Read the model definition and answer for the solid it produces. Units are mm, in the model's axes. Coordinates: 2 decimals unless noted, no trailing zeros. Loops run counter-clockwise (first coordinate to the right, second up) from the corner with the lowest first, then second, coordinate; pieces in that order, holes last. Notation, with made-up numbers: (-29, -16) - (27, -16) arc R28 ccw to (27, 3) - close; hole circle Ø7 at (-15.5, -20). An arc over 180 degrees is marked (long way). Use one line per item in the form item = value. Start each with the question number.
1) A cutting plane is placed at C-C (z = 8.5). State how many separate pieces and enclosed holes the cut face has, and give its area (3 significant figures).
2) The mould has two halves that part along Y. Classify faces 1 (the face through (153.21, 173.15, 4.93)), 2 (the face through (221.595, -27.339, 5.07)), 3 (the face through (249.34, 0.04, 4.93)): released by +Y, released by -Y, zero draft, split by the parting line, or undercut.
3) Each of these flat-tipped pins is pushed along its axis until it touches: P1, Ø5, axis at y = -71, z = 7, coming from the -X side; P2, Ø5, axis at x = 8, z = 3, coming from the +Y side; P3, Ø5, axis at y = 136.5, z = 6, coming from the -X side; P4, Ø12, axis at x = 11, y = 127.5, coming from the +Z side. Where does it stop, or does it pass through?
4) Consider line 1 (Y direction, x = 0, z = 4); line 2 (X direction, y = 32, z = 4.5); line 3 (X direction, y = 155, z = 5.5). Determine where each line is inside the solid, lowest interval first.
5) A cutting plane is placed at A-A (x = -90). Give the vertices of the cut face in (y, z), and give its area (3 significant figures).
6) A cutting plane is placed at B-B (y = -139.5). Give the vertices of the cut face in (x, z), and give its area (3 significant figures).
from build123d import *

# Parameters (mm, degrees)
ESQUISSE1_R             = 47.5
BOSS_EXTRU_1_DEPTH      = 10
ESQUISSE9_W             = 150
ESQUISSE9_H             = 120
BOSS_EXTRU_2_DEPTH      = 10
ESQUISSE10_W            = 10
ESQUISSE10_H            = 50
ESQUISSE10_W_2          = 50
ESQUISSE10_H_2          = 10
ENL_V_MAT_EXTRU_1_DEPTH = 10


with BuildPart() as part:
    # Esquisse1 → Boss.-Extru.1 (new body)
    with BuildSketch(Plane.XY):
        Polygon((-255.775862069, 10.959681362), (-205, -75.190256718), (205, -75.190256718), (255.775862069, 10.959681362), (50, 336.353741833), (-50, 336.353741833), align=None)
        with Locations((-157.5, 0)):
            Circle(ESQUISSE1_R, mode=Mode.SUBTRACT)
        with Locations((-52.5, 0)):
            Circle(ESQUISSE1_R, mode=Mode.SUBTRACT)
        with Locations((52.5, 0)):
            Circle(ESQUISSE1_R, mode=Mode.SUBTRACT)
        with Locations((157.5, 0)):
            Circle(ESQUISSE1_R, mode=Mode.SUBTRACT)
        with Locations((-105, 90.932667397)):
            Circle(ESQUISSE1_R, mode=Mode.SUBTRACT)
        with Locations((0, 90.932667397)):
            Circle(ESQUISSE1_R, mode=Mode.SUBTRACT)
        with Locations((105, 90.932667397)):
            Circle(ESQUISSE1_R, mode=Mode.SUBTRACT)
        with Locations((-52.5, 181.865334795)):
            Circle(ESQUISSE1_R, mode=Mode.SUBTRACT)
        with Locations((52.5, 181.865334795)):
            Circle(ESQUISSE1_R, mode=Mode.SUBTRACT)
        with Locations((0, 272.798002192)):
            Circle(ESQUISSE1_R, mode=Mode.SUBTRACT)
    extrude(amount=BOSS_EXTRU_1_DEPTH)

    # Esquisse9 → Boss.-Extru.2 (add)
    with BuildSketch(Plane.XY.offset(10)):
        with Locations((0, -135.190256718)):
            Rectangle(ESQUISSE9_W, ESQUISSE9_H)
    extrude(amount=-BOSS_EXTRU_2_DEPTH)

    # Esquisse10 → Enlèv. mat.-Extru.1 (cut)
    with BuildSketch(Plane.XY.offset(10)):
        with Locations((-70, -129.244737692)):
            Rectangle(ESQUISSE10_W, ESQUISSE10_H)
        with Locations((0, -190.190256718)):
            Rectangle(ESQUISSE10_W_2, ESQUISSE10_H_2)
        with Locations((-140, -70.190256718)):
            Rectangle(ESQUISSE10_W_2, ESQUISSE10_H_2)
        Polygon((-217.693965517, -53.652772198), (-209.078971709, -48.575185991), (-234.466902744, -5.500216951), (-243.081896552, -10.577803158), align=None)
        Polygon((-229.051724138, 53.218650255), (-220.599930359, 47.873822668), (-167.151654497, 132.391760453), (-175.603448276, 137.736588039), align=None)
        Polygon((-130.172413793, 209.576835156), (-121.720620015, 204.23200757), (-68.272344153, 288.749945355), (-76.724137931, 294.094772941), align=None)
        with Locations((0, 331.353741833)):
            Rectangle(ESQUISSE10_W_2, ESQUISSE10_H_2)
        Polygon((68.272344153, 288.749945355), (76.724137931, 294.094772941), (130.172413793, 209.576835156), (121.720620015, 204.23200757), align=None)
        Polygon((167.151654497, 132.391760453), (175.603448276, 137.736588039), (229.051724138, 53.218650255), (220.599930359, 47.873822668), align=None)
        Polygon((234.466902744, -5.500216951), (243.081896552, -10.577803158), (217.693965517, -53.652772198), (209.078971709, -48.575185991), align=None)
        with Locations((140, -70.190256718)):
            Rectangle(ESQUISSE10_W_2, ESQUISSE10_H_2)
        with Locations((70, -129.244737692)):
            Rectangle(ESQUISSE10_W, ESQUISSE10_H)
    extrude(amount=-ENL_V_MAT_EXTRU_1_DEPTH, mode=Mode.SUBTRACT)


solid = part.part
Found:
q1.separate_pieces = 1
q1.enclosed_holes = 10
q1.area = 78,300 mm^2
q2.face_1 = released by +Y
q2.face_2 = undercut
q2.face_3 = released by -Y
q3.P1 = -208.94
q3.P2 = 326.35
q3.P3 = -175.6
q3.P4 = through
q4.line_1 = -185.19 to 43.43, 138.43 to 225.3, 320.3 to 326.35
q4.line_2 = -242.47 to -192.6, -122.4 to -87.6, -17.4 to 17.4, 87.6 to 122.4, 192.6 to 242.47
q4.line_3 = -164.69 to -91.67, -13.33 to 13.33, 91.67 to 164.69
q5.outline = (-75.19, 0) - (-29.15, 0) - (-29.15, 10) - (-75.19, 10) - close; (29.15, 0) - (45.86, 0) - (45.86, 10) - (29.15, 10) - close; (136, 0) - (152.71, 0) - (152.71, 10) - (136, 10) - close; (211.02, 0) - (254.39, 0) - (254.39, 10) - (211.02, 10) - close
q5.area = 1,230 mm^2
q6.outline = (-65, 0) - (65, 0) - (65, 10) - (-65, 10) - close
q6.area = 1,300 mm^2
